from build123d import *

# Parameters (mm, degrees)
SKETCH1_W                = 38.1
SKETCH1_H                = 63.5
SKETCH1_R                = 4.064
BOSS_EXTRUDE1_DEPTH      = 10
BOSS_EXTRUDE2_DEPTH      = 10
BOSS_EXTRUDE2_DEPTH_BACK = 8.5
SKETCH2_R                = 1.5
SKETCH3_R                = 1.5
BOSS_EXTRUDE3_DEPTH      = 10
SKETCH2_2_R              = 1.5
CUT_EXTRUDE1_DEPTH       = 10
CUT_EXTRUDE2_START       = 10
SKETCH3_2_R              = 1.5
CUT_EXTRUDE2_DEPTH       = 10


with BuildPart() as part:
    # Sketch1 → Boss-Extrude1 (new body)
    with BuildSketch(Plane(origin=(0, 0, 0), x_dir=(1, 0, 0), z_dir=(0, 1, 0))):
        with Locations((19.05, -31.75)):
            Rectangle(SKETCH1_W, SKETCH1_H)
        with Locations(Location((19.05, -44.45, 0), (0, 0, 270))):
            Circle(SKETCH1_R, mode=Mode.SUBTRACT)
    extrude(amount=BOSS_EXTRUDE1_DEPTH)

    # Sketch2 → Boss-Extrude2 (add, two sides: drawn at the far end of the back side and taken through both)
    with BuildSketch(Plane(origin=(0, 0, 0), x_dir=(0, 0, -1), z_dir=(1, 0, 0)).offset(-BOSS_EXTRUDE2_DEPTH_BACK)):
        Polygon((-33.5, 0), (-33.5, -10), (-63.5, -10), (-63.5, 0), (-63.5, 10), (-33.5, 10), align=None)
        with Locations((-59.6, 8)):
            Circle(SKETCH2_R, mode=Mode.SUBTRACT)
        with Locations((-37.4, -2.3)):
            Circle(SKETCH2_R, mode=Mode.SUBTRACT)
    extrude(amount=BOSS_EXTRUDE2_DEPTH + BOSS_EXTRUDE2_DEPTH_BACK)

    # Sketch3 → Boss-Extrude3 (add)
    with BuildSketch(Plane.XY):
        Polygon((13.25, -21), (13.25, -3), (16.25, -3), (16.25, -21), (38.1, -21), (38.1, 10), (0, 10), (0, -21), align=None)
        with Locations((4.75, -16)):
            Circle(SKETCH3_R, mode=Mode.SUBTRACT)
        with Locations((24.75, -16)):
            Circle(SKETCH3_R, mode=Mode.SUBTRACT)
        with Locations((4.75, 4)):
            Circle(SKETCH3_R, mode=Mode.SUBTRACT)
        with Locations((24.75, 4)):
            Circle(SKETCH3_R, mode=Mode.SUBTRACT)
    extrude(amount=-BOSS_EXTRUDE3_DEPTH)

    # Sketch2_2 → Cut-Extrude1 (cut)
    with BuildSketch(Plane(origin=(0, 0, 0), x_dir=(0, 0, -1), z_dir=(1, 0, 0))):
        with Locations((-59.6, 8)):
            Circle(SKETCH2_2_R)
    extrude(amount=CUT_EXTRUDE1_DEPTH, mode=Mode.SUBTRACT)

    # Sketch3_2 → Cut-Extrude2 (cut)
    with BuildSketch(Plane.XY.offset(CUT_EXTRUDE2_START)):
        with Locations((24.75, 4)):
            Circle(SKETCH3_2_R)
        with Locations((4.75, 4)):
            Circle(SKETCH3_2_R)
    extrude(amount=-CUT_EXTRUDE2_DEPTH, mode=Mode.SUBTRACT)


solid = part.part
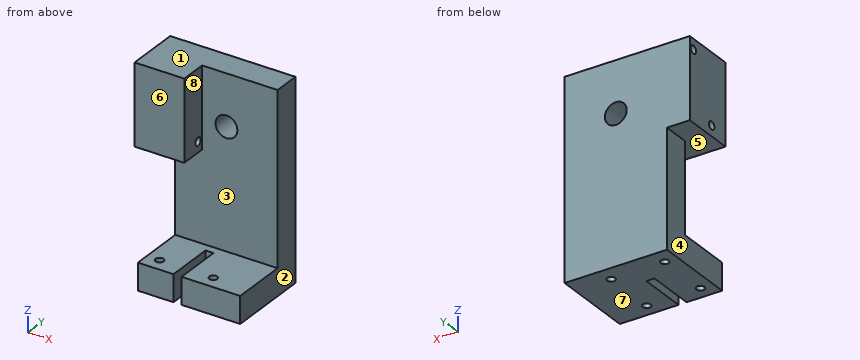
Work out the finished part from the listing and answer in its coordinate system (mm). Face numbers are marked on the shaded views. A direction names the side the tool comes from. Round coordinates to 2 decimals unless told otherwise and drop trailing zeros. Write each loop counter-clockwise with the first axis right and the second up, starting at its lowest first coordinate (ties: lowest second). Pieces come first, ordered by that corner, then holes. Notation, with made-up numbers: (75.5, 24) - (124.5, 24) arc R11 cw to (124.5, 40) - close; hole circle Ø9 at (11.5, 36.5). An arc over 180 degrees is marked (long way). Answer in a Markdown table with one row per item. Add a question column.
1. A cutting plane is placed at B-B, the plane z = 44.45. Determine the outline of the cut face in (x, y).
2. Given pin 1 (6 mm diameter, centred on x = 26, z = 50.5, fed in from -Y); pin 2 (12 mm diameter, centred on x = 14, z = 54, fed in from -Y); pin 3 (1 mm diameter, centred on x = 12.5, y = -10.5, fed in from +Z), each flat-ended and moving along its own axis, determine where each tip first touches the part or whether it passes through.
3. Find the intervals of material crossed by line 1 along Y through (x, z) = (4.75, -3.5); line 2 along X through (y, z) = (5.5, 44.45); line 3 along Y through (x, z) = (4, -7), in increasing order. Write a range as from..to.
4. The mould has two halves that part along Z. Classify the marked faces 1, 2 and 3: +Z half, -Z half, draft (parallel to the pull), parting line (faces both ways), or undercut.
5. For the marked faces 4, 5, 6, 7 and 8, determine the directions among +Z, -Z, +X, -X, +Y, -Y from which every point of the face is accessible in a straight line to the end or side of a thin tool.
6. A cutting plane is placed at A-A, the plane x = 4.75. Determine the outline of the cut face in (y, z), and give its area (3 significant figures).
7. A cutting plane is placed at C-C, the plane y = 4. Determine the outline of the cut face in (x, z), and give its area (3 significant figures).
8. A cutting plane is placed at D-D, the plane x = -4. Determine the outline of the cut face in (y, z).
Worked out:
| question | item | result |
|---|---|---|
| 1 | outline | (-8.5, -10) - (10, -10) - (10, 0) - (14.99, 0) - (14.99, 10) - (-8.5, 10) - close; (23.11, 0) - (38.1, 0) - (38.1, 10) - (23.11, 10) - close |
| 2 | pin 1 | y = 0 |
| 2 | pin 2 | y = -10 |
| 2 | pin 3 | z = 0 |
| 3 | line 1 | -21..-17.5, -14.5..2.5, 5.5..10 |
| 3 | line 2 | -8.5..14.99, 23.11..38.1 |
| 3 | line 3 | -21..-17.3, -14.7..2.7, 5.3..10 |
| 4 | face 1 | +Z half |
| 4 | face 2 | draft |
| 4 | face 3 | undercut |
| 5 | face 4 | -Z, -X, +Y, -Y |
| 5 | face 5 | -X, -Y |
| 5 | face 6 | +Z, +X, -X, -Y |
| 5 | face 7 | -Z, +X, -X, +Y, -Y |
| 5 | face 8 | +Z, +X, -Y |
| 6 | outline | (-21, -10) - (-17.5, -10) - (-17.5, 0) - (-21, 0) - close; (-14.5, -10) - (2.5, -10) - (2.5, 10) - (5.5, 10) - (5.5, -10) - (10, -10) - (10, 63.5) - (-10, 63.5) - (-10, 33.5) - (0, 33.5) - (0, 0) - (-14.5, 0) - close; hole circle Ø3 at (-2.3, 37.4); hole circle Ø3 at (8, 59.6) |
| 6 | area | 1,140 mm^2 |
| 7 | outline | (-8.5, 33.5) - (0, 33.5) - (0, -10) - (3.25, -10) - (3.25, 10) - (6.25, 10) - (6.25, -10) - (23.25, -10) - (23.25, 10) - (26.25, 10) - (26.25, -10) - (38.1, -10) - (38.1, 63.5) - (-8.5, 63.5) - close; hole circle Ø8.13 at (19.05, 44.45) |
| 7 | area | 2,880 mm^2 |
| 8 | outline | (-10, 33.5) - (10, 33.5) - (10, 63.5) - (-10, 63.5) - close; hole circle Ø3 at (-2.3, 37.4); hole circle Ø3 at (8, 59.6) |
